Could you check a few things on this model? Use its own coordinates, in mm. A direction names the side the tool comes from. Round coordinates to 2 decimals unless told otherwise and drop trailing zeros. Order: outer loops, then holes, each group sorted by start corner. A loop starts at its lowest first (then second) coordinate and runs counter-clockwise, first axis right, second up. Notation, with made-up numbers: (-13.75, 71) - (34.25, 71) arc R10 ccw to (34.25, 83) - close; hole circle Ø9 at (6.5, -13). An arc over 180 degrees is marked (long way). Use one line per item in the form item = value.
from build123d import *

# Parameters (mm, degrees)
SM_BASE_FLANGE_1_DEPTH = 160
CUT_EXTRUDE_2_DEPTH    = 174.583553368
CUT_EXTRUDE_3_REACH    = 175.943
OTHER_1_DEPTH          = 2.5
OTHER_1_2_DEPTH        = 2.5


# Read off the part's stored shape, not the designer's step: 断开-边角1
# Sheet-metal steps are written as plain solids
with BuildPart() as part:
    # Sketch 1 → 基体-法兰1 (new, symmetric)
    with BuildSketch(Plane(origin=(0, 0, 0), x_dir=(0, 0, -1), z_dir=(1, 0, 0))):
        with BuildLine():
            Line((-60, 0), (-4.5, 0))
            ThreePointArc((-4.5, 0), (-1.318019485, 1.318019485), (0, 4.5))
            Line((0, 4.5), (0, 35))
            Line((0, 35), (-2.5, 35))
            Line((-2.5, 35), (-2.5, 4.5))
            ThreePointArc((-2.5, 4.5), (-3.085786438, 3.085786438), (-4.5, 2.5))
            Line((-4.5, 2.5), (-60, 2.5))
            Line((-60, 2.5), (-60, 0))
        make_face()
    extrude(amount=SM_BASE_FLANGE_1_DEPTH, both=True)

    # 草图5 → 切除-拉伸2 (cut, through all)
    with BuildSketch(Plane.XY.offset(2.5)):
        with BuildLine():
            Line((-115.5, 25), (-115.5, 15))
            ThreePointArc((-115.5, 15), (-120, 10.5), (-124.5, 15))
            Line((-124.5, 15), (-124.5, 25))
            ThreePointArc((-124.5, 25), (-120, 29.5), (-115.5, 25))
        make_face()
        with BuildLine():
            Line((115.5, 25), (115.5, 15))
            ThreePointArc((115.5, 15), (120, 10.5), (124.5, 15))
            Line((124.5, 15), (124.5, 25))
            ThreePointArc((124.5, 25), (120, 29.5), (115.5, 25))
        make_face()
        with BuildLine():
            Line((4.5, 25), (4.5, 15))
            ThreePointArc((4.5, 15), (0, 10.5), (-4.5, 15))
            Line((-4.5, 15), (-4.5, 25))
            ThreePointArc((-4.5, 25), (0, 29.5), (4.5, 25))
        make_face()
    extrude(amount=-CUT_EXTRUDE_2_DEPTH, mode=Mode.SUBTRACT)

    # 草图6 → 切除-拉伸3 (cut, up to next)
    with BuildSketch(Plane(origin=(0, 2.5, 0), x_dir=(1, 0, 0), z_dir=(0, 1, 0)), mode=Mode.PRIVATE) as cut_extrude_3_sk1:
        with BuildLine():
            ThreePointArc((-19.874276789, -24.875176049), (-84.173281176, -30.783424559), (-147.390129564, -43.932547934))
            ThreePointArc((-147.390129564, -43.932547934), (-149.865003298, -48.219154984), (-145.578396248, -50.694028718))
            ThreePointArc((-145.578396248, -50.694028718), (-83.138615298, -37.706535603), (-19.629980312, -31.870911838))
            ThreePointArc((-19.629980312, -31.870911838), (-16.254260656, -28.250895705), (-19.874276789, -24.875176049))
        make_face()
    cut_extrude_3_tool1 = extrude(cut_extrude_3_sk1.sketch, amount=-CUT_EXTRUDE_3_REACH, mode=Mode.PRIVATE) & part.part
    # 草图6 → 切除-拉伸3 (cut, up to next)
    with BuildSketch(Plane(origin=(0, 2.5, 0), x_dir=(1, 0, 0), z_dir=(0, 1, 0)), mode=Mode.PRIVATE) as cut_extrude_3_sk2:
        with BuildLine():
            ThreePointArc((19.874276789, -24.875176049), (84.173281176, -30.783424559), (147.390129564, -43.932547934))
            ThreePointArc((147.390129564, -43.932547934), (149.865003298, -48.219154984), (145.578396248, -50.694028718))
            ThreePointArc((145.578396248, -50.694028718), (83.138615298, -37.706535603), (19.629980312, -31.870911838))
            ThreePointArc((19.629980312, -31.870911838), (16.254260656, -28.250895705), (19.874276789, -24.875176049))
        make_face()
    cut_extrude_3_tool2 = extrude(cut_extrude_3_sk2.sketch, amount=-CUT_EXTRUDE_3_REACH, mode=Mode.PRIVATE) & part.part
    add(cut_extrude_3_tool1.solids().sort_by_distance((-83.461905, 2.5, 35.543351))[0], mode=Mode.SUBTRACT)
    add(cut_extrude_3_tool2.solids().sort_by_distance((83.461905, 2.5, 35.543351))[0], mode=Mode.SUBTRACT)

    # Other 1 outline → Other 1 (cut)
    with BuildSketch(Plane(origin=(0, 0, 0), x_dir=(1, 0, 0), z_dir=(0, 1, 0))):
        with BuildLine():
            Line((-160, -60), (-158, -60))
            ThreePointArc((-158, -60), (-159.414213562, -59.414213562), (-160, -58))
            Line((-160, -58), (-160, -60))
        make_face()
        with BuildLine():
            ThreePointArc((160, -58), (159.414213562, -59.414213562), (158, -60))
            Line((158, -60), (160, -60))
            Line((160, -60), (160, -58))
        make_face()
    extrude(amount=OTHER_1_DEPTH, mode=Mode.SUBTRACT)

    # Other 1 2 outline → Other 1 2 (cut)
    with BuildSketch(Plane.XY):
        with BuildLine():
            Line((160, 35), (158, 35))
            ThreePointArc((158, 35), (159.414213562, 34.414213562), (160, 33))
            Line((160, 33), (160, 35))
        make_face()
        with BuildLine():
            ThreePointArc((-160, 33), (-159.414213562, 34.414213562), (-158, 35))
            Line((-158, 35), (-160, 35))
            Line((-160, 35), (-160, 33))
        make_face()
    extrude(amount=OTHER_1_2_DEPTH, mode=Mode.SUBTRACT)


solid = part.part
Item 1: Will these pins go through, and if not, where does the flat tip stop? P1, Ø10, axis at x = 112.5, z = 13.5, coming from the -Y side; P2, Ø5, axis at x = 45.5, z = 25, coming from the +Y side.
Found:
P1 = 0
P2 = 2.5
Item 2: Imagine slicing it at A-A on y = 20.5. Please give me the cut outline in (x, z), plus the area to 4 significant figures.
Found:
outline = (-160, 0) - (-124.5, 0) - (-124.5, 2.5) - (-160, 2.5) - close; (-115.5, 0) - (-4.5, 0) - (-4.5, 2.5) - (-115.5, 2.5) - close; (4.5, 0) - (115.5, 0) - (115.5, 2.5) - (4.5, 2.5) - close; (124.5, 0) - (160, 0) - (160, 2.5) - (124.5, 2.5) - close
area = 732.5 mm2
Item 3: Imagine slicing it at B-B on x = 30.5. Please give me the cut outline in (y, z), plus the area to 3 significant figures.
Found:
outline = (0, 4.5) arc R4.5 ccw to (4.5, 0) - (35, 0) - (35, 2.5) - (4.5, 2.5) arc R2 cw to (2.5, 4.5) - (2.5, 25.35) - (0, 25.35) - close; (0, 32.36) - (2.5, 32.36) - (2.5, 60) - (0, 60) - close
area = 210 mm2
Item 4: Imagine slicing it at C-C on x = 120. Please give me the cut outline in (y, z).
Found:
outline = (0, 4.5) arc R4.5 ccw to (4.5, 0) - (10.5, 0) - (10.5, 2.5) - (4.5, 2.5) arc R2 cw to (2.5, 4.5) - (2.5, 37.32) - (0, 37.32) - close; (0, 44.48) - (2.5, 44.48) - (2.5, 60) - (0, 60) - close; (29.5, 0) - (35, 0) - (35, 2.5) - (29.5, 2.5) - close
Item 5: If we mould it in two halves opening along Z, with no side actions, what happens to faces 1 (the face through (83.28, 1.27, 30.65)), 2 (the face through (2, 9, 0)), 3 (the face through (2, 30, 2.5)), 4 (the face through (2, 0, 33))? For each: released by +Z, released by -Z, zero draft, split by the parting line, or undercut.
Found:
face_1 = undercut
face_2 = released by -Z
face_3 = released by +Z
face_4 = zero draft
Item 6: Imagine slicing it at D-D on x = -121. Please give me the cut outline in (y, z).
Found:
outline = (0, 4.5) arc R4.5 ccw to (4.5, 0) - (10.61, 0) - (10.61, 2.5) - (4.5, 2.5) arc R2 cw to (2.5, 4.5) - (2.5, 37.53) - (0, 37.53) - close; (0, 44.7) - (2.5, 44.7) - (2.5, 60) - (0, 60) - close; (29.39, 0) - (35, 0) - (35, 2.5) - (29.39, 2.5) - close
Item 7: I need wall thicknesses on L1, parallel to Z at x = 7, y = 10.5; L2, parallel to Z at x = 13, y = 3. Which ranges of each line are inside material? Lowest first, please.
Found:
L1 = 0 to 2.5
L2 = 0.26 to 3.18
Item 8: For faces 5 (the face through (2, 2.5, 32)), 6 (the face through (160, 2, 21)), 7 (the face through (-83.28, 1.27, 30.65)), which set-ups out of +Z, -Z, +X, -X, +Y, -Y let a thin tool reach every point of the face, with its end or its side?
Found:
face_5 = +Z, +X, -X, +Y
face_6 = +Z, -Z, +X, +Y, -Y
face_7 = +Y, -Y
